Input: part model. Units: mm. Frame: model coordinates. A direction names the side the tool comes from. Coordinates: 2 decimals unless noted, no trailing zeros. Loops run counter-clockwise (first coordinate to the right, second up) from the corner with the lowest first, then second, coordinate; pieces in that order, holes last.
(1) Section A-A, the plane z = 15. Return loops of the section in (x, y).
(2) Contact query for flat-ended pins moving along their axis: P1, Ø5, axis at x = -7.5, z = 24.5, coming from the -Y side; P2, Ø5, axis at x = 28, z = 0, coming from the +Y side; P3, Ø2.5, axis at x = 7.5, z = 24.5, coming from the +Y side. Output: stop coordinate, or through.
(3) Section B-B, the plane y = 1.2. Give the number of separate pieces and of enclosed holes in the cut face, then the cut area to 3 significant figures.
(4) Line query: L1, parallel to X at y = 2.45, z = -25; L2, parallel to Z at x = 0, y = 0.45; L3, parallel to Z at x = -7.5, y = 1.35. Output: solid intervals per line, ascending.
(5) Section C-C, the plane x = 28. Return loops of the section in (y, z).
(6) Mould query, pull axis X, two halves, no side actions, for faces 1 (the face through (-0.391, 2.507, 38.026)), 2 (the face through (31.4, 1.48, -44.43)), 3 (the face through (0, 1, -45)). Classes: released by +X, released by -X, zero draft, split by the parting line, or undercut.
(7) Section D-D, the plane x = -7.5. Return loops of the section in (y, z), then the cut area to 3 significant figures.
(8) Set-up query: faces 4 (the face through (-1.315, 1.521, 4.986)), 5 (the face through (29.3, 2, 1.3)). Return all of +Z, -Z, +X, -X, +Y, -Y with unobstructed straight access to the full face (end or side cutting, diameter ignored); none if empty.
Autodesk Inventor part; units mm, degrees
ref_plane "YZ Plane" through (0, 0, 0) normal (1, 0, 0) x (0, 1, 0)
ref_plane "XZ Plane" through (0, 0, 0) normal (0, 1, 0) x (-1, 0, 0)
ref_plane "XY Plane" through (0, 0, 0) normal (0, 0, 1) x (1, 0, 0)
sketch "Sketch1" plane through (0, 0, 0) normal (0, 1, 0) x (-1, 0, 0)
  line L0 (-30, -43) -> (30, -43)
  line L1 (30, -43) -> (30, 43)
  line L2 (30, 43) -> (-30, 43)
  line L3 (-30, 43) -> (-30, -43)
  line L4 (-30, -43) -> (30, 43) construction
  line L5 (30, -43) -> (-30, 43) construction
  line L6 (0, 43) -> (0, 45)
  line L7 (30, 0) -> (32, 0)
  line L8 (-30, -45) -> (30, -45)
  line L9 (32, -43) -> (32, 43)
  line L10 (30, 45) -> (-30, 45)
  line L11 (-32, 43) -> (-32, -43)
  line L12 (-32, -45) -> (32, 45) construction
  line L13 (32, -45) -> (-32, 45) construction
  arc A0 (-32, -43) -> (-30, -45) centre (-30, -43) ccw
  arc A1 (30, -45) -> (32, -43) centre (30, -43) ccw
  arc A2 (32, 43) -> (30, 45) centre (30, 43) ccw
  arc A3 (-30, 45) -> (-32, 43) centre (-30, 43) ccw
  point P0 (0, 0)
  point P1 (0, 0)
  dimension "d4" = 60
  dimension "d5" = 86
  dimension "d6" = 2
  dimension "d7" = 2
  dimension "d8" = 2
extrude "Extrusion1" add sketch "Sketch1" along normal blind 3
sketch "Sketch2" plane through (0, 3, 0) normal (0, 1, 0) x (1, 0, 0)
  circle A0 centre (0, 41) radius 1.5
  circle A1 centre (-28, 0) radius 1.5
  circle A2 centre (0, -41) radius 1.5
  circle A3 centre (28, 0) radius 1.5
  line L0 (-32, 43) -> (-32, -43)
  arc A4 (-32, -43) -> (-30, -45) centre (-30, -43) ccw
  line L1 (-30, -45) -> (30, -45)
  arc A5 (-30, 45) -> (-32, 43) centre (-30, 43) ccw
  line L2 (30, 45) -> (-30, 45)
  arc A6 (32, 43) -> (30, 45) centre (30, 43) ccw
  line L3 (32, -43) -> (32, 43)
  arc A7 (30, -45) -> (32, -43) centre (30, -43) ccw
  circle A8 centre (-20, 25) radius 2
  circle A9 centre (7.5, 2.5) radius 1.6
  circle A10 centre (7.5, -24.5) radius 1.6
  circle A11 centre (0, -15) radius 10.1
  circle A12 centre (-7.5, 2.5) radius 1.6
  circle A13 centre (-7.5, -24.5) radius 1.6
  line L4 (0, 0) -> (0, 4.1)
  circle A14 centre (20, 25) radius 5
  point P0 (-5.5, -13.5)
  dimension "d11" = 4
  dimension "d13" = 20.2
  dimension "d14" = 3.2
  dimension "d15" = 3.2
  dimension "d16" = 3.2
  dimension "d17" = 3.2
  dimension "d20" = 10
extrude "Extrusion2" cut sketch "Sketch2" against normal through all contours A0 | A1 | A2 | A3 | A8 | A9 | A10 | A11 | A12 | A13 | A14
sketch "Sketch3" plane through (0, 3, 0) normal (0, 1, 0) x (1, 0, 0)
  circle A0 centre (-28, 0) radius 1.5
  circle A1 centre (0, 41) radius 1.5
  circle A2 centre (0, -41) radius 1.5
  circle A3 centre (28, 0) radius 1.5
  circle A4 centre (0, -41) radius 3
  circle A5 centre (-28, 0) radius 3
  circle A6 centre (0, 41) radius 3
  circle A7 centre (28, 0) radius 3
  point P0 (0, 0)
  dimension "d21" = 6
  dimension "d22" = 6
  dimension "d23" = 6
  dimension "d24" = 6
extrude "Extrusion3" cut sketch "Sketch3" against normal blind 1
properties part number "Case Top"
Report:
1. outline: (-32, 0) - (-10.1, 0) - (-10.1, 3) - (-32, 3) - close; (10.1, 0) - (32, 0) - (32, 3) - (10.1, 3) - close
2. P1: stops at y = 0
2. P2: stops at y = 2
2. P3: passes through
3. separate pieces: 1
3. enclosed holes: 11
3. area: 5,280 mm2
4. L1: x = -32 to -22, -18 to 15, 25 to 32
4. L2: z = -45 to -42.5, -39.5 to 4.9, 25.1 to 39.5, 42.5 to 45
4. L3: z = -45 to -4.1, -0.9 to 8.24, 21.76 to 22.9, 26.1 to 45
5. outline: (0, -45) - (3, -45) - (3, -3) - (2, -3) - (2, -1.5) - (0, -1.5) - close; (0, 1.5) - (2, 1.5) - (2, 3) - (3, 3) - (3, 45) - (0, 45) - close
6. face 1: undercut
6. face 2: released by +X
6. face 3: zero draft
7. outline: (0, -45) - (3, -45) - (3, -4.1) - (0, -4.1) - close; (0, -0.9) - (3, -0.9) - (3, 8.24) - (0, 8.24) - close; (0, 21.76) - (3, 21.76) - (3, 22.9) - (0, 22.9) - close; (0, 26.1) - (3, 26.1) - (3, 45) - (0, 45) - close
7. area: 210 mm2
8. face 4: +Y, -Y
8. face 5: +Y
